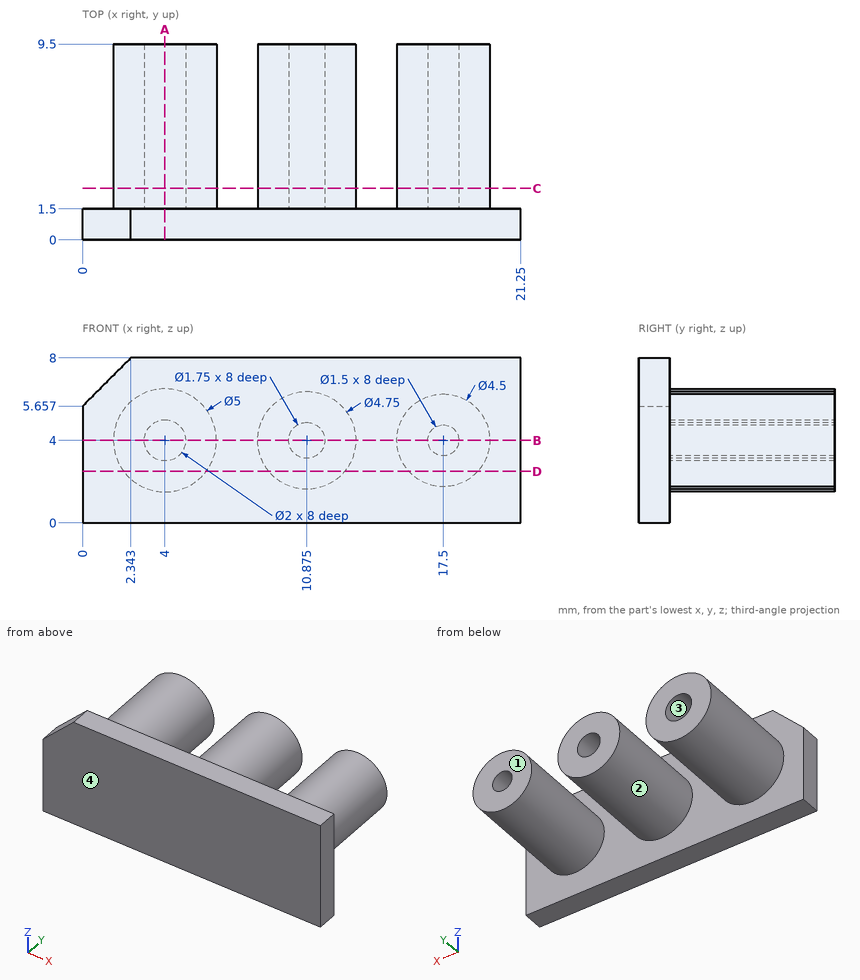
Drawing for the job (mm, zero at the part's lowest x, y, z). A direction names the side the tool comes from. Round coordinates to 2 decimals unless told otherwise and drop trailing zeros. Write each loop counter-clockwise with the first axis right and the second up, starting at its lowest first coordinate (ties: lowest second). Pieces come first, ordered by that corner, then holes.
Item 1: Drop flat-ended pins along their axis: pin 1 Ø0.6 at (x, z) = (3.5, 4) entering from +Y; pin 2 Ø3 at (x, y) = (17.5, 8) entering from +Z. Give the stop position or say it passes through.
Filled in:
pin 1: stops at y = 1.5
pin 2: stops at z = 6.25
Item 2: Band-saw the part on D-D on z = 2.5. Write the cut outline in (x, y), then the cut area to 3 significant figures.
Filled in:
outline: (0, 0) - (21.25, 0) - (21.25, 1.5) - (19.18, 1.5) - (19.18, 9.5) - (15.82, 9.5) - (15.82, 1.5) - (12.72, 1.5) - (12.72, 9.5) - (9.03, 9.5) - (9.03, 1.5) - (6, 1.5) - (6, 9.5) - (2, 9.5) - (2, 1.5) - (0, 1.5) - close
area: 120 mm2
Item 3: Drill centre lines: L1, parallel to X at y = 6, z = 4; L2, parallel to Z at x = 11.5, y = 7; L3, parallel to Y at x = 1, z = 2.25. Where is each one in solid material? Low to high.
Filled in:
L1: x = 1.5 to 3, 5 to 6.5, 8.5 to 10, 11.75 to 13.25, 15.25 to 16.75, 18.25 to 19.75
L2: z = 1.71 to 3.39, 4.61 to 6.29
L3: y = 0 to 1.5
Item 4: Band-saw the part on C-C on y = 2.5. Write the cut outline in (x, z) (3 decimals).
Filled in:
outline: circle Ø5 at (4, 4); circle Ø4.75 at (10.875, 4); circle Ø4.5 at (17.5, 4); hole circle Ø2 at (4, 4); hole circle Ø1.75 at (10.875, 4); hole circle Ø1.5 at (17.5, 4)
Item 5: Tool access for the marked faces 3 and 4: list every direction of +Z, -Z, +X, -X, +Y, -Y with a clear straight run to the whole face (end or side of a thin tool).
Filled in:
face 3: +Y
face 4: +Z, -Z, +X, -X, -Y
Item 6: Band-saw the part on B-B on z = 4. Write the cut outline in (x, y).
Filled in:
outline: (0, 0) - (21.25, 0) - (21.25, 1.5) - (19.75, 1.5) - (19.75, 9.5) - (18.25, 9.5) - (18.25, 1.5) - (16.75, 1.5) - (16.75, 9.5) - (15.25, 9.5) - (15.25, 1.5) - (13.25, 1.5) - (13.25, 9.5) - (11.75, 9.5) - (11.75, 1.5) - (10, 1.5) - (10, 9.5) - (8.5, 9.5) - (8.5, 1.5) - (6.5, 1.5) - (6.5, 9.5) - (5, 9.5) - (5, 1.5) - (3, 1.5) - (3, 9.5) - (1.5, 9.5) - (1.5, 1.5) - (0, 1.5) - close
Item 7: Mould opens along X. For the marked faces 1 and 2 say: released by +X, released by -X, zero draft, split by the parting line, or undercut.
Filled in:
face 1: zero draft
face 2: undercut
Item 8: Band-saw the part on A-A on x = 4. Write the cut outline in (y, z), then the cut area to 3 significant figures.
Filled in:
outline: (0, 0) - (1.5, 0) - (1.5, 1.5) - (9.5, 1.5) - (9.5, 3) - (1.5, 3) - (1.5, 5) - (9.5, 5) - (9.5, 6.5) - (1.5, 6.5) - (1.5, 8) - (0, 8) - close
area: 36.0 mm2
